Read the model definition and answer for the solid it produces. Units are mm, in the model's axes. Round coordinates to 2 decimals unless told otherwise and drop trailing zeros. Order: outer loops, then holes, each group sorted by start corner. A loop starts at its lowest first (then second) coordinate and runs counter-clockwise, first axis right, second up. Notation, with made-up numbers: (32, 3) - (58, 3) arc R30 cw to (58, 37) - close; hole circle Ø7 at (-22, 62). An arc over 180 degrees is marked (long way). One line per question, with ' | ' between items. Start each with the question number.
1) The part is cut by section B-B, the plane z = 20.5. Give the vertices of the cut face in (x, y), plus the area to 3 significant figures.
2) Flat-ended cylindrical pins translate along their axes: pin 1 (8 mm diameter, centred on y = -179, z = 5, fed in from +X); pin 2 (1 mm diameter, centred on x = -290, y = -248, fed in from -Z); pin 3 (3 mm diameter, centred on y = -445, z = 7.5, fed in from +X). Find the tip coordinate at first contact, or state that the pin passes through.
3) Straight lines are drawn through the part: line 1 (X direction, y = 42, z = 23.5); line 2 (X direction, y = -345, z = 16.75). For each, find the intervals that lie inside material, in ascending order. Write a range as from..to.
from build123d import *

# Parameters (mm, degrees)
F0_W     = 660.4
F0_H     = 762
F1_DEPTH = 25.4
F2_SIZE  = 25.39999


# Not quite as in the source:
# - a fillet or chamfer is up to 0.001 mm smaller than in the source, because OpenCascade refuses the exact size


with BuildPart() as f1:
    # F0 (on Top) → F1 (new body)
    with BuildSketch(Plane.XY):
        with Locations((-148.2397035837, -222.647351265)):
            Rectangle(F0_W, F0_H)
    extrude(amount=F1_DEPTH)

    # F2 (size 25.4 in the source; OpenCascade refuses exactly that, so slightly less here)
    f2_edges = [f1.edges().sort_by_distance(p)[0] for p in [
        (181.960296, -222.647351, 25.4),
    ]]
    chamfer(f2_edges, length=F2_SIZE)


solid = f1.part
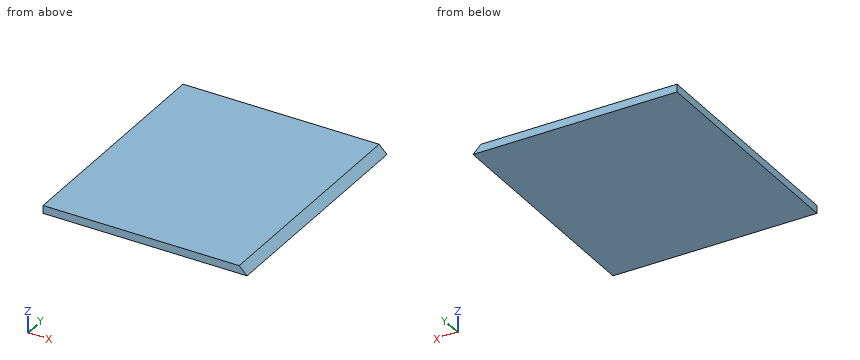
Values:
1) outline: (-478.44, -603.65) - (161.46, -603.65) - (161.46, 158.35) - (-478.44, 158.35) - close | area: 488,000 mm^2
2) pin 1: stops at x = 180.96 | pin 2: stops at z = 0 | pin 3: stops at x = 175.96
3) line 1: x = -478.44..158.46 | line 2: x = -478.44..165.21
